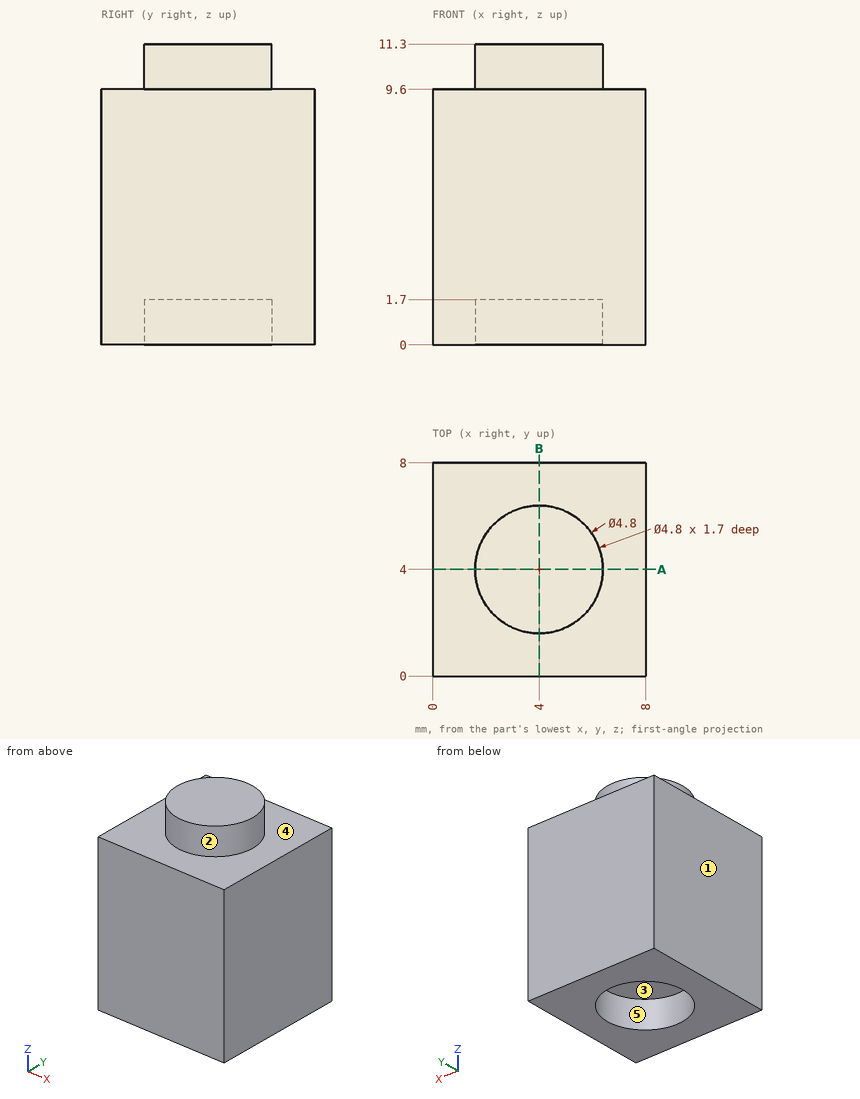
Study the drawing (mm; zero at the part's minimum x, y, z) and answer. A direction names the side the tool comes from. Give positions to 0.01 mm unless a question says otherwise; leave off trailing zeros. Order: outer loops, then holes, each group sorted by start corner. A loop starts at its lowest first (then second) coordinate and runs counter-clockwise, first axis right, second up. Notation, with made-up numbers: (25, -33.5) - (30, -33.5) arc R9 cw to (30, -21.5) - close; hole circle Ø7 at (22, -37.75). An arc over 180 degrees is marked (long way). Answer as CSV lines item,"result". Start each with the question number.
Q1. For the marked faces 1 and 2, determine the directions among +Z, -Z, +X, -X, +Y, -Y from which every point of the face is accessible in a straight line to the end or side of a thin tool.
Q2. The part is cut by section A-A (y = 4). Write down the section's boundary in (x, z), then the cut area to 3 significant figures.
Q3. Find the intervals of material crossed by L1, parallel to Z at x = 1, y = 6; L2, parallel to Y at x = 4, z = 1.3; L3, parallel to X at y = 4, z = 10.5, in increasing order. Write a range as [from, to].
Q4. The mould has two halves that part along Z. Classify the marked faces 3, 4 and 5: +Z half, -Z half, draft (parallel to the pull), parting line (faces both ways), or undercut.
Q5. Given pin 1 Ø3 at (y, z) = (1, 7) entering from -X, flat-ended and moving along its own axis, determine where the tip first touches the part or whether it passes through.
Check result:
1,face 1,"+Z, -Z, -X, +Y, -Y"
1,face 2,"+Z"
2,outline,"(0, 0) - (1.6, 0) - (1.6, 1.7) - (6.4, 1.7) - (6.4, 0) - (8, 0) - (8, 9.6) - (6.4, 9.6) - (6.4, 11.3) - (1.6, 11.3) - (1.6, 9.6) - (0, 9.6) - close"
2,area,"76.8 mm²"
3,L1,"z = [0, 9.6]"
3,L2,"y = [0, 1.6], [6.4, 8]"
3,L3,"x = [1.6, 6.4]"
4,face 3,"-Z half"
4,face 4,"+Z half"
4,face 5,"draft"
5,pin 1,"stops at x = 0"
